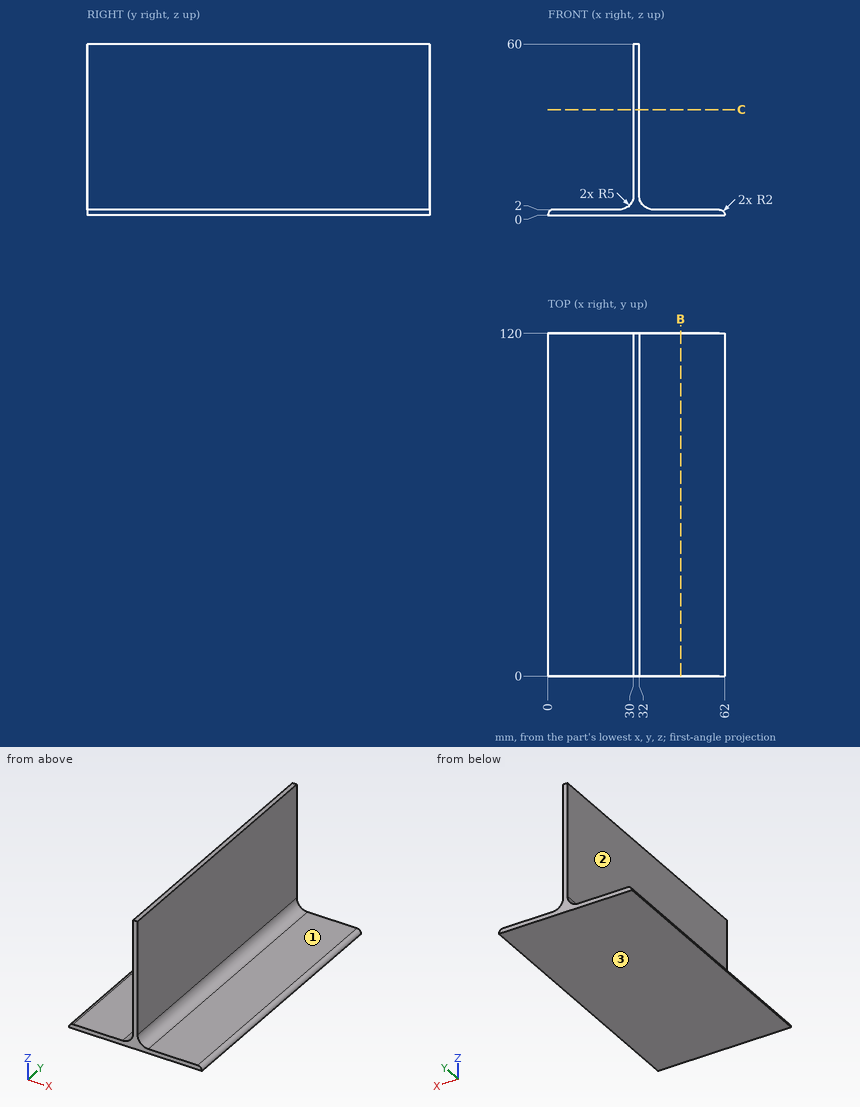
Job drawing, mm, ordinate dimensions from the low corner. One solid piece. A direction names the side the tool comes from. Give positions to 0.01 mm unless a question says otherwise; leave off trailing zeros. Loops run counter-clockwise (first coordinate to the right, second up) from the corner with the lowest first, then second, coordinate; pieces in that order, holes last. Notation, with made-up numbers: (55, -13) - (66, -13) arc R33 cw to (66, 18) - close; hole circle Ø4 at (27, 74.25). An arc over 180 degrees is marked (long way). Use one line per item in the form item = value.
(1) 3-axis set-ups, long thin cutter, end or side, ignore diameter. For the marked faces 1, 2 and 3: which of +Z, -Z, +X, -X, +Y, -Y reach the whole face in a straight line?
Determined:
face_1 = +Z, +X, +Y, -Y
face_2 = +Z, -X, +Y, -Y
face_3 = -Z, +X, -X, +Y, -Y
(2) Cut at B-B (x = 46.5). Give the cut face in (y, z).
Determined:
outline = (0, 0) - (120, 0) - (120, 2) - (0, 2) - close
(3) Cut at C-C (z = 37). Give the cut face in (x, y), then the cut area to 3 significant figures.
Determined:
outline = (30, 0) - (32, 0) - (32, 120) - (30, 120) - close
area = 240 mm^2
(4) Drill centre lines: L1, parallel to X at y = 34, z = 23; L2, parallel to Z at x = 25, y = 27.5; L3, parallel to Z at x = 33.5, y = 14.5. Where is each one in solid material? Low to high.
Determined:
L1 = 30 to 32
L2 = 0 to 2
L3 = 0 to 3.43
(5) Drop flat-ended pins along their axis: P1, Ø18.5, axis at x = 43, y = 88.5, coming from the +Z side; P2, Ø12, axis at x = 16, y = 50, coming from the -Z side; P3, Ø3, axis at y = 46.5, z = 38.5, coming from the -X side; P4, Ø16, axis at y = 55.5, z = 23, coming from the +X side. Give the stop position or say it passes through.
Determined:
P1 = 3.2
P2 = 0
P3 = 30
P4 = 32
